```python
from build123d import *

# Parameters (mm, degrees)
SKETCH1_W           = 28.5
SKETCH1_H           = 28.5
BOSS_EXTRUDE1_DEPTH = 7
FILLET1_R           = 2
SKETCH2_R           = 11
BOSS_EXTRUDE2_DEPTH = 1.6
SKETCH3_R           = 4
CUT_EXTRUDE1_DEPTH  = 1.6
SKETCH6_W           = 28.2
SKETCH6_H           = 28.2
BOSS_EXTRUDE4_DEPTH = 14
FILLET2_R           = 2
SKETCH7_W           = 28.5
SKETCH7_H           = 28.5
BOSS_EXTRUDE5_DEPTH = 7
FILLET3_R           = 2
SKETCH9_R           = 1.4
CUT_EXTRUDE3_DEPTH  = 42.7
SKETCH10_R          = 3.5
CUT_EXTRUDE4_DEPTH  = 4
FILLET4_R           = 0.5
FILLET5_R           = 0.5
CUT_EXTRUDE5_START  = -0.1
SKETCH11_R          = 12
SKETCH11_R_2        = 11
CUT_EXTRUDE5_DEPTH  = 0.1
CUT_EXTRUDE6_START  = -2.5
SKETCH12_R          = 4
CUT_EXTRUDE6_DEPTH  = 2.5
SKETCH13_R          = 2.5
BOSS_EXTRUDE7_DEPTH = 0.5
FILLET6_R           = 0.2
SKETCH_1_R          = 3
SHAFT_DEPTH         = 148


with BuildPart() as part:
    # Sketch1 → Boss-Extrude1 (new body)
    with BuildSketch(Plane.XY):
        Rectangle(SKETCH1_W, SKETCH1_H)
    extrude(amount=BOSS_EXTRUDE1_DEPTH)

    # Fillet1
    fillet1_edges = [part.edges().sort_by_distance(p)[0] for p in [
        (14.25, -14.25, 3.5),
        (-14.25, -14.25, 3.5),
        (-14.25, 14.25, 3.5),
        (14.25, 14.25, 3.5),
    ]]
    fillet(fillet1_edges, radius=FILLET1_R)

    # Sketch2 → Boss-Extrude2 (add)
    with BuildSketch(Plane.XY.offset(7)):
        Circle(SKETCH2_R)
    extrude(amount=BOSS_EXTRUDE2_DEPTH)

    # Sketch3 → Cut-Extrude1 (cut)
    with BuildSketch(Plane.XY.offset(8.6)):
        Circle(SKETCH3_R)
    extrude(amount=-CUT_EXTRUDE1_DEPTH, mode=Mode.SUBTRACT)

    # Sketch6 → Boss-Extrude4 (add)
    with BuildSketch(Plane(origin=(0, 0, 0), x_dir=(-1, 0, 0), z_dir=(0, 0, -1))):
        Rectangle(SKETCH6_W, SKETCH6_H)
    extrude(amount=BOSS_EXTRUDE4_DEPTH)

    # Fillet2
    # the kernel refuses this fillet: 2 mm, written as the material it takes off along each edge
    with BuildSketch(Plane(origin=(-14.1, -14.1, 0), x_dir=(0, 1, 0), z_dir=(0, 0, -1)), Plane(origin=(-14.1, 14.1, 0), x_dir=(1, 0, 0), z_dir=(0, 0, -1))) as fillet2_piece_1:
        with BuildLine():
            CenterArc((FILLET2_R, FILLET2_R), FILLET2_R, 180, 90)
            Line((0, FILLET2_R), (0, 0))
            Line((0, 0), (FILLET2_R, 0))
        make_face()
    extrude(amount=19, mode=Mode.SUBTRACT)
    with BuildSketch(Plane(origin=(14.1, 14.1, 0), x_dir=(-1, 0, 0), z_dir=(0, 0, -1)), Plane(origin=(14.1, -14.1, 0), x_dir=(0, 1, 0), z_dir=(0, 0, -1))) as fillet2_piece_2:
        with BuildLine():
            CenterArc((FILLET2_R, -FILLET2_R), FILLET2_R, 90, 90)
            Line((0, -FILLET2_R), (0, 0))
            Line((0, 0), (FILLET2_R, 0))
        make_face()
    extrude(amount=19, mode=Mode.SUBTRACT)

    # Sketch7 → Boss-Extrude5 (add)
    with BuildSketch(Plane(origin=(0, 0, -14), x_dir=(-1, 0, 0), z_dir=(0, 0, -1))):
        Rectangle(SKETCH7_W, SKETCH7_H)
    extrude(amount=BOSS_EXTRUDE5_DEPTH)

    # Fillet3
    fillet3_edges = [part.edges().sort_by_distance(p)[0] for p in [
        (-14.25, -14.25, -17.5),
        (-14.25, 14.25, -17.5),
        (14.25, 14.25, -17.5),
        (14.25, -14.25, -17.5),
    ]]
    fillet(fillet3_edges, radius=FILLET3_R)

    # Sketch9 → Cut-Extrude3 (cut)
    with BuildSketch(Plane.XY.offset(7)):
        with Locations((-11.5, 11.5)):
            Circle(SKETCH9_R)
        with Locations((11.5, 11.5)):
            Circle(SKETCH9_R)
        with Locations((11.5, -11.5)):
            Circle(SKETCH9_R)
        with Locations((-11.5, -11.5)):
            Circle(SKETCH9_R)
    extrude(amount=-CUT_EXTRUDE3_DEPTH, mode=Mode.SUBTRACT)

    # Sketch10 → Cut-Extrude4 (cut)
    with BuildSketch(Plane(origin=(0, 0, -21), x_dir=(-1, 0, 0), z_dir=(0, 0, -1))):
        with Locations((-11.5, 11.5)):
            Circle(SKETCH10_R)
        with Locations((11.5, 11.5)):
            Circle(SKETCH10_R)
        with Locations((11.5, -11.5)):
            Circle(SKETCH10_R)
        with Locations((-11.5, -11.5)):
            Circle(SKETCH10_R)
    extrude(amount=-CUT_EXTRUDE4_DEPTH, mode=Mode.SUBTRACT)

    # Fillet4
    fillet4_edges = [part.edges().sort_by_distance(p)[0] for p in [
        (14.25, -9.334936491, -19),
        (9.334936491, -14.25, -19),
        (-14.25, -9.334936491, -19),
        (-9.334936491, -14.25, -19),
        (-14.25, 9.334936491, -19),
        (-9.334936491, 14.25, -19),
        (9.334936491, 14.25, -19),
        (14.25, 9.334936491, -19),
    ]]
    fillet(fillet4_edges, radius=FILLET4_R)

    # Fillet5
    fillet5_edges = [part.edges().sort_by_distance(p)[0] for p in [
        (-14.25, 0, -21),
        (9.025126266, -9.025126266, -21),
        (0, -14.25, -21),
        (-9.025126266, -9.025126266, -21),
        (-9.025126266, 9.025126266, -21),
        (0, 14.25, -21),
        (9.025126266, 9.025126266, -21),
        (14.25, 0, -21),
        (13.983853587, 8.634752599, -21),
        (8.634752599, 13.983853587, -21),
        (13.983853587, -8.634752599, -21),
        (8.634752599, -13.983853587, -21),
        (-8.634752599, -13.983853587, -21),
        (-13.983853587, -8.634752599, -21),
        (-8.634752599, 13.983853587, -21),
        (-13.983853587, 8.634752599, -21),
    ]]
    fillet(fillet5_edges, radius=FILLET5_R)

    # Sketch11 → Cut-Extrude5 (cut)
    with BuildSketch(Plane.XY.offset(7).offset(CUT_EXTRUDE5_START)):
        Circle(SKETCH11_R)
        Circle(SKETCH11_R_2, mode=Mode.SUBTRACT)
    extrude(amount=CUT_EXTRUDE5_DEPTH, mode=Mode.SUBTRACT)

    # Sketch12 → Cut-Extrude6 (cut)
    with BuildSketch(Plane(origin=(0, 0, -21), x_dir=(-1, 0, 0), z_dir=(0, 0, -1)).offset(CUT_EXTRUDE6_START)):
        with Locations(Location((0, 0, 0), (0, 0, 180))):
            Circle(SKETCH12_R)
    extrude(amount=CUT_EXTRUDE6_DEPTH, mode=Mode.SUBTRACT)

    # Sketch13 → Boss-Extrude7 (add)
    with BuildSketch(Plane(origin=(0, 0, -18.5), x_dir=(-1, 0, 0), z_dir=(0, 0, -1))):
        Circle(SKETCH13_R)
    extrude(amount=BOSS_EXTRUDE7_DEPTH)

    # Fillet6
    fillet6_edges = [part.edges().sort_by_distance(p)[0] for p in [
        (2.5, 0, -19),
    ]]
    fillet(fillet6_edges, radius=FILLET6_R)

    # Эскиз1 → Shaft (add)
    with BuildSketch(Plane.XY.offset(7)):
        Circle(SKETCH_1_R)
    extrude(amount=SHAFT_DEPTH)


solid = part.part
```
The listing builds one solid part. Answer for the finished solid, in the listing's coordinates (mm). A direction names the side the tool comes from. Round coordinates to 2 decimals unless told otherwise and drop trailing zeros. Order: outer loops, then holes, each group sorted by start corner. A loop starts at its lowest first (then second) coordinate and runs counter-clockwise, first axis right, second up. Notation, with made-up numbers: (3.5, -20) - (39.5, -20) arc R26 cw to (39.5, 17) - close; hole circle Ø2 at (32, 43.25). An arc over 180 degrees is marked (long way). Put each result on its own line as item: value. Start each with the question number.
(1) For faces 4 (the flat face through (14.25, 0, 3)), 5 (the cylindrical face through (-9.07, -8.98, -18.77)), 6 (the cylindrical face through (-0.867, -3.905, 7.811)), 7 (the flat face through (-14.1, 0, -7)), 8 (the flat face through (14.1, 0, -7)), determine the directions among +Z, -Z, +X, -X, +Y, -Y from which every point of the face is accessible in a straight line to the end or side of a thin tool.
(2) Find section B-B (z = 61.5). Give the vertices of the cut face in (x, y).
(3) Given P1, Ø10, axis at x = 0.5, z = 81, coming from the -Y side; P2, Ø1.9, axis at x = 11, y = 10.5, coming from the -Z side; P3, Ø12, axis at x = 6.5, y = 0.5, coming from the +Z side; P4, Ø5, axis at y = 1, z = 86, coming from the -X side, each flat-ended and moving along its own axis, determine where each tip first touches the part or whether it passes through.
(4) Straight lines are drawn through the part: probe 1 along Y at (x, z) = (0, 7.5); probe 2 along Y at (x, z) = (11.5, -0.25); probe 3 along Z at (x, y) = (-11.75, -3). For each, find the intervals that lie inside material, in ascending order. Write a range as from..to.
(5) Find section A-A (x = -5.5). Give the vertices of the cut face in (y, z).
(6) Determine the mould class of faces 1 (the flat face through (-14.25, 0, -17)), 2 (the cylindrical face through (-0.867, 3.905, -19.732)), 3 (the flat face through (0, -5, 8.6)) for opening direction X: released by +X, released by -X, zero draft, split by the parting line, or undercut.
(7) Find section C-C (x = 6). Give the vertices of the cut face in (y, z).
Reply:
1. face 4: +Z, -Z, +X, +Y, -Y
1. face 5: -Z
1. face 6: +Z
1. face 7: -X, +Y, -Y
1. face 8: +X, +Y, -Y
2. outline: circle Ø6 at (0, 0)
3. P1: y = -3
3. P2: z = -17
3. P3: z = 155
3. P4: x = -3
4. probe 1: -11..-4, -3..3, 4..11
4. probe 2: -14.1..-12.9, -10.1..10.1, 12.9..14.1
4. probe 3: -21..7
5. outline: (-14.25, -20.5) arc R0.5 ccw to (-13.75, -21) - (13.75, -21) arc R0.5 ccw to (14.25, -20.5) - (14.25, -14) - (14.1, -14) - (14.1, 0) - (14.25, 0) - (14.25, 7) - (10.67, 7) - (10.67, 6.9) - (9.53, 6.9) - (9.53, 8.6) - (-9.53, 8.6) - (-9.53, 6.9) - (-10.67, 6.9) - (-10.67, 7) - (-14.25, 7) - (-14.25, 0) - (-14.1, 0) - (-14.1, -14) - (-14.25, -14) - close
6. face 1: released by -X
6. face 2: undercut
6. face 3: zero draft
7. outline: (-14.25, -20.5) arc R0.5 ccw to (-13.75, -21) - (13.75, -21) arc R0.5 ccw to (14.25, -20.5) - (14.25, -14) - (14.1, -14) - (14.1, 0) - (14.25, 0) - (14.25, 7) - (10.39, 7) - (10.39, 6.9) - (9.22, 6.9) - (9.22, 8.6) - (-9.22, 8.6) - (-9.22, 6.9) - (-10.39, 6.9) - (-10.39, 7) - (-14.25, 7) - (-14.25, 0) - (-14.1, 0) - (-14.1, -14) - (-14.25, -14) - close
